Geometry check sheet. Reference: the model listing, model coordinates, mm. A direction names the side the tool comes from. Round coordinates to 2 decimals unless told otherwise and drop trailing zeros. Write each loop counter-clockwise with the first axis right and the second up, starting at its lowest first coordinate (ties: lowest second). Pieces come first, ordered by that corner, then holes. Notation, with made-up numbers: M -29,2.25 L 12,2.25 A20 ccw 12,23.25 Z; hole C -22,74.25 d9. An arc over 180 degrees is marked long. Put each result on its own line as item: value. Start each with the question number.
(1) Tool access check on faces 1 (the flat face through (-35, 5, 5)), 2 (the flat face through (25, 10, 15)), 3 (the flat face through (5, 0.3, 19.9)), 4 (the flat face through (-15, -15, 5)). Record the directions out of +Z, -Z, +X, -X, +Y, -Y that give a thin tool (end or side, any length) a straight path to the whole face; none if there is none.
(2) Gauge pin test, flat ends, axial feed: pin 1 (11.5 mm diameter, centred on x = -20, y = 5, fed in from +Z); pin 2 (10 mm diameter, centred on y = -16.5, z = 3, fed in from -X); pin 3 (10 mm diameter, centred on x = 27.5, z = 20.5, fed in from -Y). Record the tip position at first contact, or that the pin passes through.
(3) Section check D-D on y = -14.5. Record the cut outline in (x, z).
(4) Section check B-B on z = 20. Record the cut outline in (x, y).
(5) Mould release check, pull along Y, two halves, no side actions. Record for faces 5 (the flat face through (-25, -10.881, 5)), 6 (the flat face through (8, 20, 11)), 7 (the cylindrical face through (10.07, -6.08, 15.12)): pulls with the +Y half, pulls with the -Y half, needs draft (parallel to the pull), parting line crosses it, or undercut.
(6) Material ranges on probe 1 along Y at (x, z) = (-20, 6.25); probe 2 along Z at (x, y) = (12.25, -5); probe 3 along X at (y, z) = (18, 19), recorded low to high.
(7) Section check C-C on x = -20. Record the cut outline in (y, z), then the cut area to 3 significant figures.
(8) Section check A-A on y = -8. Record the cut outline in (x, z).
from build123d import *

# Parameters (mm, degrees)
F1_DEPTH = 10
F2_DEPTH = 30
F3_R     = 5
F4_DEPTH = 25
F5_R     = 5
F6_DEPTH = 25


with BuildPart() as f1:
    # F0 (on Top) → F1 (new body)
    with BuildSketch(Plane.XY):
        Polygon((5, -20), (5, 20), (-35, 20), (-35, -10.881234), (-15, -10.881234), (-15, -20), align=None)
    extrude(amount=F1_DEPTH)

    # F0 (on Top) → F2 (join)
    with BuildSketch(Plane.XY):
        Polygon((35, 10), (35, 20), (15, 20), (5, 20), (5, -20), (15, -20), (15, 10), align=None)
    extrude(amount=F2_DEPTH)

    # F3 (on face) → F4 (cut)
    with BuildSketch(Plane.YZ.offset(15)):
        with Locations((-5, 20)):
            Circle(F3_R)
    extrude(amount=-F4_DEPTH, mode=Mode.SUBTRACT)

    # F5 (on face) → F6 (cut)
    with BuildSketch(Plane.XY.offset(10)):
        with Locations((-20, 5)):
            Circle(F5_R)
    extrude(amount=-F6_DEPTH, mode=Mode.SUBTRACT)


solid = f1.part
Answers follow:
1. face 1: +Z, -Z, -X, +Y, -Y
1. face 2: +Z, -Z, +X, -Y
1. face 3: +Z, -X, +Y, -Y
1. face 4: +Z, -Z, -X, -Y
2. pin 1: stops at z = 10
2. pin 2: stops at x = -15
2. pin 3: stops at y = 10
3. outline: M -15,0 L 15,0 L 15,30 L 5,30 L 5,10 L -15,10 Z
4. outline: M 5,-20 L 15,-20 L 15,-10 L 5,-10 Z; M 5,0 L 15,0 L 15,10 L 35,10 L 35,20 L 5,20 Z
5. face 5: pulls with the -Y half
5. face 6: pulls with the +Y half
5. face 7: undercut
6. probe 1: y = -10.88 to 0, 10 to 20
6. probe 2: z = 0 to 15, 25 to 30
6. probe 3: x = 5 to 35
7. outline: M -10.88,0 L 0,0 L 0,10 L -10.88,10 Z; M 10,0 L 20,0 L 20,10 L 10,10 Z
7. area: 209 mm^2
8. outline: M -35,0 L 15,0 L 15,16 L 5,16 L 5,10 L -35,10 Z; M 5,24 L 15,24 L 15,30 L 5,30 Z
